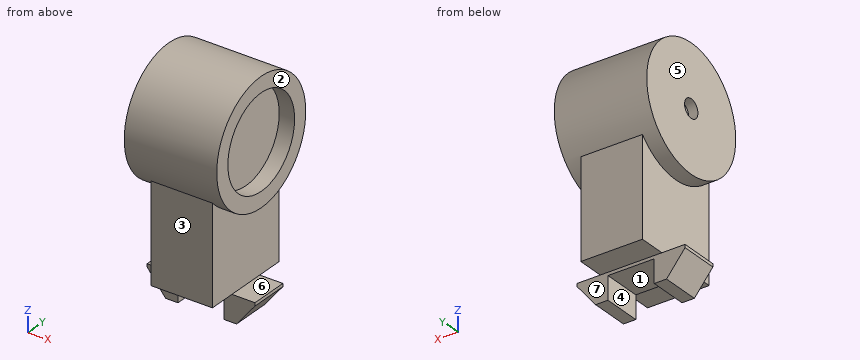
```python
from build123d import *

# Parameters (mm, degrees)
SKETCH1_R           = 40
BOSS_EXTRUDE1_DEPTH = 60
BOSS_EXTRUDE3_REACH = 132.133
SKETCH2_W           = 40
SKETCH2_H           = 60
SKETCH3_W           = 70
SKETCH3_H           = 25
BOSS_EXTRUDE4_DEPTH = 2
BOSS_EXTRUDE5_DEPTH = 25
SKETCH8_R           = 30
CUT_EXTRUDE3_DEPTH  = 10
SKETCH9_R           = 6
CUT_EXTRUDE4_DEPTH  = 6


with BuildPart() as part:
    # Sketch1 → Boss-Extrude1 (new body)
    with BuildSketch(Plane(origin=(0, 0, 0), x_dir=(0, 0, -1), z_dir=(1, 0, 0))):
        Circle(SKETCH1_R)
    extrude(amount=BOSS_EXTRUDE1_DEPTH)

    # Sketch2 → Boss-Extrude3 (add, up to next)
    with BuildSketch(Plane.XY.offset(-90.13280569), mode=Mode.PRIVATE) as boss_extrude3_sk1:
        with Locations((30, 0)):
            Rectangle(SKETCH2_W, SKETCH2_H)
    boss_extrude3_tool1 = extrude(boss_extrude3_sk1.sketch, amount=BOSS_EXTRUDE3_REACH, mode=Mode.PRIVATE) - part.part
    add(boss_extrude3_tool1.solids().sort_by_distance((30, 0, -90.132806))[0])

    # Sketch3 → Boss-Extrude4 (add)
    with BuildSketch(Plane(origin=(0, 0, -90.13280569), x_dir=(-1, 0, 0), z_dir=(0, 0, -1))):
        with Locations((-30, 0)):
            Rectangle(SKETCH3_W, SKETCH3_H)
    extrude(amount=BOSS_EXTRUDE4_DEPTH)

    # Sketch5 → Boss-Extrude5 (add)
    with BuildSketch(Plane(origin=(0, 12.5, 0), x_dir=(1, 0, 0), z_dir=(0, 1, 0))):
        Polygon((-5, 92.13280569), (7, 107.13280569), (15, 107.13280569), (15, 92.13280569), align=None)
        Polygon((45, 107.13280569), (45, 92.13280569), (65, 92.13280569), (53, 107.13280569), align=None)
    extrude(amount=-BOSS_EXTRUDE5_DEPTH)

    # Sketch8 → Cut-Extrude3 (cut)
    with BuildSketch(Plane(origin=(60, 0, 0), x_dir=(0, 0, -1), z_dir=(1, 0, 0))):
        Circle(SKETCH8_R)
    extrude(amount=-CUT_EXTRUDE3_DEPTH, mode=Mode.SUBTRACT)

    # Sketch9 → Cut-Extrude4 (cut)
    with BuildSketch(Plane.ZY):
        Circle(SKETCH9_R)
    extrude(amount=-CUT_EXTRUDE4_DEPTH, mode=Mode.SUBTRACT)


solid = part.part
```
Check sheet for the modelled part. Datum: model origin and axes. Units: mm. Face numbers are marked on the shaded views. A direction names the side the tool comes from. Coordinates: 2 decimals unless noted, no trailing zeros. Loops run counter-clockwise (first coordinate to the right, second up) from the corner with the lowest first, then second, coordinate; pieces in that order, holes last.
1) Gauge pin test, flat ends, axial feed: pin 1 (6 mm diameter, centred on x = 16.5, y = 1, fed in from -Z); pin 2 (9 mm diameter, centred on x = 39.5, y = 23.5, fed in from -Z); pin 3 (6 mm diameter, centred on x = 22, y = -26, fed in from +Z); pin 4 (1.5 mm diameter, centred on x = 26, z = -86, fed in from -Y). Record the tip position at first contact, or that the pin passes through.
2) Sectioned sample at B-B (x = 36). Record the boundary of the cut face in (y, z), and give its area (3 significant figures).
3) Sectioned sample at D-D (z = -95). Record the boundary of the cut face in (x, y).
4) Sectioned sample at C-C (z = 0). Record the boundary of the cut face in (x, y).
5) Material ranges on probe 1 along Y at (x, z) = (56, 0); probe 2 along X at (y, z) = (12.5, -53); probe 3 along X at (y, z) = (-19, 33), recorded low to high.
6) Release check for a two-part mould opening along X. For the marked faces 1, 2 and 3 record: released by +X, released by -X, zero draft, split by the parting line, or undercut.
7) Sectioned sample at A-A (y = 0). Record the boundary of the cut face in (x, z).
8) Access from +Z, -Z, +X, -X, +Y, -Y to the whole of each face (thin tool, end or side, straight path). Record for the marked faces 4, 5, 6 and 7.
Check sheet entries:
1. pin 1: stops at z = -107.13
1. pin 2: stops at z = -90.13
1. pin 3: stops at z = 32.73
1. pin 4: stops at y = -30
2. outline: (-30, -90.13) - (-12.5, -90.13) - (-12.5, -92.13) - (12.5, -92.13) - (12.5, -90.13) - (30, -90.13) - (30, -26.46) arc R40 ccw (long way) to (-30, -26.46) - close
2. area: 8,330 mm2
3. outline: (-2.71, -12.5) - (15, -12.5) - (15, 12.5) - (-2.71, 12.5) - close; (45, -12.5) - (62.71, -12.5) - (62.71, 12.5) - (45, 12.5) - close
4. outline: (0, -40) - (60, -40) - (60, -30) - (50, -30) - (50, 30) - (60, 30) - (60, 40) - (0, 40) - (0, 6) - (6, 6) - (6, -6) - (0, -6) - close
5. probe 1: y = -40 to -30, 30 to 40
5. probe 2: x = 10 to 50
5. probe 3: x = 0 to 60
6. face 1: undercut
6. face 2: released by +X
6. face 3: zero draft
7. outline: (-5, -92.13) - (7, -107.13) - (15, -107.13) - (15, -92.13) - (45, -92.13) - (45, -107.13) - (53, -107.13) - (65, -92.13) - (65, -90.13) - (50, -90.13) - (50, -40) - (60, -40) - (60, -30) - (50, -30) - (50, 30) - (60, 30) - (60, 40) - (0, 40) - (0, 6) - (6, 6) - (6, -6) - (0, -6) - (0, -40) - (10, -40) - (10, -90.13) - (-5, -90.13) - close
8. face 4: -Z, +Y, -Y
8. face 5: +Z, -X, +Y, -Y
8. face 6: +X, +Y, -Y
8. face 7: -Z, +X, -X, +Y
